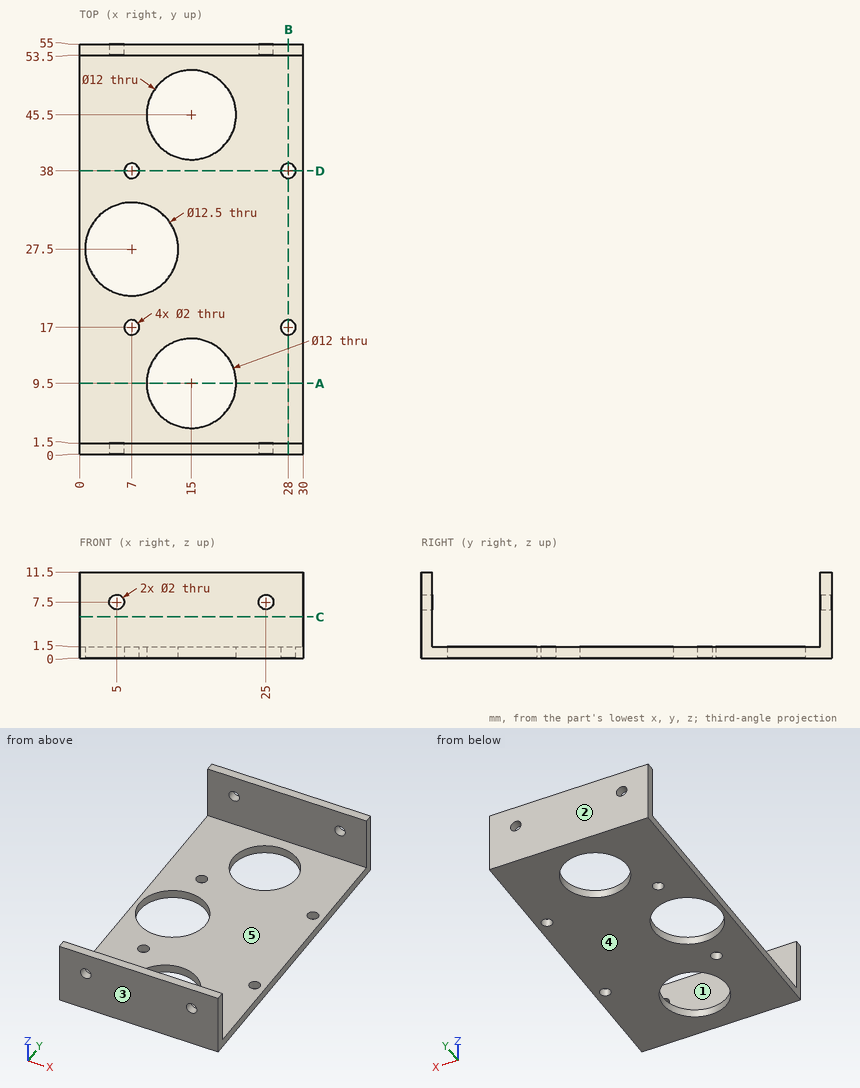
Part print with two shaded views. Sizes in mm from the minimum x, y, z corner. A direction names the side the tool comes from. Give positions to 0.01 mm unless a question says otherwise; leave off trailing zeros. Order: outer loops, then holes, each group sorted by start corner. A loop starts at its lowest first (then second) coordinate and runs counter-clockwise, first axis right, second up. Notation, with made-up numbers: M 39,70.5 L 91,70.5 A18 cw 91,90.5 Z; hole C -9,-23.5 d7. An arc over 180 degrees is marked long. Use one line per item in the form item = value.
1) Saw through at D-D (y = 38). Give the cut face in (x, z), plus the area to 3 significant figures.
Calculated:
outline = M 0,0 L 6,0 L 6,1.5 L 0,1.5 Z; M 8,0 L 27,0 L 27,1.5 L 8,1.5 Z; M 29,0 L 30,0 L 30,1.5 L 29,1.5 Z
area = 39.0 mm2
2) Probe probe 1 along X at (y, z) = (38, 1.1); probe 2 along Y at (x, z) = (28, 1.2); probe 3 along Y at (x, z) = (17.25, 4.5). List the from-to ranges inside material, lowest first.
Calculated:
probe_1 = 0 to 6, 8 to 27, 29 to 30
probe_2 = 0 to 16, 18 to 37, 39 to 55
probe_3 = 0 to 1.5, 53.5 to 55
3) Two-plate mould, pull along Y, no slides. Class the marked faces 3, 4 and 5: released by +Y, released by -Y, zero draft, split by the parting line, or undercut.
Calculated:
face_3 = released by -Y
face_4 = zero draft
face_5 = undercut
4) Drop flat-ended pins along their axis: pin 1 (1.2 mm diameter, centred on x = 5, z = 7.5, fed in from -Y); pin 2 (14 mm diameter, centred on x = 15, y = 45.5, fed in from +Z). Give the stop position or say it passes through.
Calculated:
pin_1 = through
pin_2 = 1.5
5) Tool access for the marked faces 1 and 2: list every direction of +Z, -Z, +X, -X, +Y, -Y with a clear straight run to the whole face (end or side of a thin tool).
Calculated:
face_1 = +Z, +X, -X
face_2 = +Z, -Z, +X, -X, +Y
6) Saw through at B-B (x = 28). Give the cut face in (y, z).
Calculated:
outline = M 0,0 L 16,0 L 16,1.5 L 1.5,1.5 L 1.5,11.5 L 0,11.5 Z; M 18,0 L 37,0 L 37,1.5 L 18,1.5 Z; M 39,0 L 55,0 L 55,11.5 L 53.5,11.5 L 53.5,1.5 L 39,1.5 Z
7) Saw through at A-A (y = 9.5). Give the cut face in (x, z), plus the area to 3 significant figures.
Calculated:
outline = M 0,0 L 9,0 L 9,1.5 L 0,1.5 Z; M 21,0 L 30,0 L 30,1.5 L 21,1.5 Z
area = 27.0 mm2
8) Saw through at C-C (z = 5.5). Give the cut face in (x, y), plus the area to 3 significant figures.
Calculated:
outline = M 0,0 L 30,0 L 30,1.5 L 0,1.5 Z; M 0,53.5 L 30,53.5 L 30,55 L 0,55 Z
area = 90.0 mm2
